Part print with two shaded views. Sizes in mm from the minimum x, y, z corner. A direction names the side the tool comes from. Give positions to 0.01 mm unless a question says otherwise; leave off trailing zeros. Write each loop counter-clockwise with the first axis right and the second up, starting at its lowest first coordinate (ties: lowest second). Pieces come first, ordered by that corner, then holes.
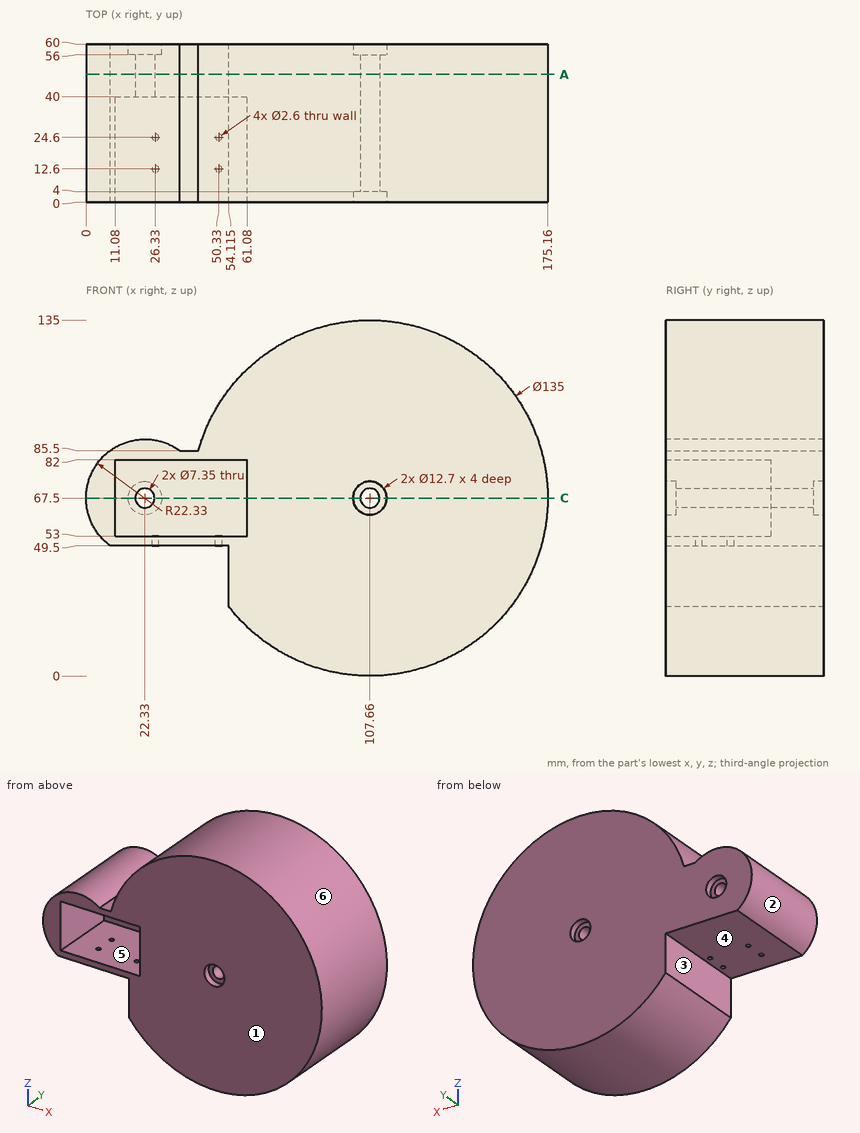
1) Mould opens along X. For the marked faces 1, 2 and 3 say: +X half, -X half, draft (parallel to the pull), parting line (faces both ways), or undercut.
Check result:
face 1: draft
face 2: undercut
face 3: -X half
2) Saw through at C-C (z = 67.5). Write the cut outline in (x, y) (1 decimal), and give its area (3 significant figures).
Check result:
outline: (0, 0) - (11.1, 0) - (11.1, 40) - (18.7, 40) - (18.7, 56) - (16, 56) - (16, 60) - (0, 60) - close; (26, 40) - (61.1, 40) - (61.1, 0) - (101.3, 0) - (101.3, 4) - (104, 4) - (104, 56) - (101.3, 56) - (101.3, 60) - (28.7, 60) - (28.7, 56) - (26, 56) - close; (111.3, 4) - (114, 4) - (114, 0) - (175.2, 0) - (175.2, 60) - (114, 60) - (114, 56) - (111.3, 56) - close
area: 7,860 mm2
3) Saw through at A-A (y = 48.5). State how many separate pieces and enclosed holes the cut face has, and give its area (3 significant figures).
Check result:
separate pieces: 1
enclosed holes: 2
area: 15,500 mm2
4) 3-axis set-ups, long thin cutter, end or side, ignore diameter. For the marked faces 4, 5 and 6: which of +Z, -Z, +X, -X, +Y, -Y reach the whole face in a straight line?
Check result:
face 4: -Z, -X, +Y, -Y
face 5: -Y
face 6: +Y, -Y
5) Flat gauge pins, fed straight in: P1, Ø10, axis at y = 21.5, z = 58.5, coming from the +X side; P2, Ø1.6, axis at x = 26.33, y = 12.6, coming from the -Z side; P3, Ø1.5, axis at x = 58, y = 19, coming from the -Z side; P4, Ø10, axis at x = 109.5, z = 65.5, coming from the +Y side. Where does each tip first touch, or does it go through?
Check result:
P1: stops at x = 175.04
P2: stops at z = 82
P3: stops at z = 20.98
P4: stops at y = 60
6) Drill centre lines: L1, parallel to X at y = 57, z = 67 (1 decimal); L2, parallel to Y at x = 32, z = 61.5; L3, parallel to Z at x = 46, y = 39.5 (1 decimal). Where is each one in solid material? Low to high.
Check result:
L1: x = 0 to 16, 28.7 to 101.3, 114 to 175.2
L2: y = 40 to 60
L3: z = 49.5 to 53, 82 to 95
